Part model, mm, in its own coordinate system. A direction names the side the tool comes from. Round coordinates to 2 decimals unless told otherwise and drop trailing zeros. Write each loop counter-clockwise with the first axis right and the second up, starting at its lowest first coordinate (ties: lowest second). Pieces come first, ordered by that corner, then holes. Notation, with made-up numbers: (-20, 30.5) -> (12, 30.5) arc R7 ccw to (12, 36.5) -> close; hole circle Ø4 at (81, 41.25). An arc over 180 degrees is marked (long way). Return JSON: item names as keys, results as strings. Group by question number.
```python
from build123d import *

# Parameters (mm, degrees)
BASE_FLANGE1_DEPTH = 600
EDGE_FLANGE1_DEPTH = 1200
SKETCH7_R          = 4
CUT_EXTRUDE1_DEPTH = 10


# Sheet-metal steps are written as plain solids
with BuildPart() as part:
    # Sketch1 → Base-Flange1 (new, symmetric)
    with BuildSketch(Plane(origin=(0, 0, 0), x_dir=(0, 0, -1), z_dir=(1, 0, 0))):
        with BuildLine():
            Line((0, 0), (0, -299.494103784))
            ThreePointArc((0, -299.494103784), (0.129412109, -299.911119881), (0.47217601, -300.181606158))
            Line((0.47217601, -300.181606158), (649.872346171, -549.950902374))
            ThreePointArc((649.872346171, -549.950902374), (650.002298395, -549.987621585), (650.136770161, -550))
            Line((650.136770161, -550), (950, -550))
            Line((950, -550), (950, -552))
            Line((950, -552), (650.136717071, -552))
            ThreePointArc((650.136717071, -552), (649.637152182, -551.954006147), (649.154377846, -551.817589676))
            Line((649.154377846, -551.817589676), (-0.245782148, -302.04829737))
            ThreePointArc((-0.245782148, -302.04829737), (-1.519211001, -301.043392746), (-2, -299.494103784))
            Line((-2, -299.494103784), (-2, 0))
            Line((-2, 0), (0, 0))
        make_face()
    extrude(amount=BASE_FLANGE1_DEPTH, both=True)

    # Edge-Flange1 section (across the edge) → Edge-Flange1 (add)
    with BuildSketch(Plane(origin=(600, 0.7366, 2), x_dir=(0, -1, 0), z_dir=(-1, 0, 0))):
        with BuildLine():
            Line((-2, 0.7366), (-2, 33))
            Line((-2, 33), (0, 33))
            Line((0, 33), (0, 0.7366))
            ThreePointArc((0, 0.7366), (0.215745145, 0.215745145), (0.7366, 0))
            Line((0.7366, 0), (0.7366, -2))
            ThreePointArc((0.7366, -2), (-1.198468417, -1.198468417), (-2, 0.7366))
        make_face()
    extrude(amount=EDGE_FLANGE1_DEPTH)

    # Sketch7 → Cut-Extrude1 (cut)
    with BuildSketch(Plane.XZ.offset(-0.7366)):
        with Locations(Location((-550, 18.8683, 0), (0, 0, 270))):
            Circle(SKETCH7_R)
        with Locations(Location((-450, 18.8683, 0), (0, 0, 270))):
            Circle(SKETCH7_R)
        with Locations(Location((-350, 18.8683, 0), (0, 0, 270))):
            Circle(SKETCH7_R)
        with Locations(Location((-250, 18.8683, 0), (0, 0, 270))):
            Circle(SKETCH7_R)
        with Locations(Location((-150, 18.8683, 0), (0, 0, 270))):
            Circle(SKETCH7_R)
        with Locations(Location((-50, 18.8683, 0), (0, 0, 270))):
            Circle(SKETCH7_R)
        with Locations(Location((50, 18.8683, 0), (0, 0, 270))):
            Circle(SKETCH7_R)
        with Locations(Location((150, 18.8683, 0), (0, 0, 270))):
            Circle(SKETCH7_R)
        with Locations(Location((250, 18.8683, 0), (0, 0, 270))):
            Circle(SKETCH7_R)
        with Locations(Location((350, 18.8683, 0), (0, 0, 270))):
            Circle(SKETCH7_R)
        with Locations(Location((450, 18.8683, 0), (0, 0, 270))):
            Circle(SKETCH7_R)
        with Locations(Location((550, 18.8683, 0), (0, 0, 270))):
            Circle(SKETCH7_R)
    extrude(amount=-CUT_EXTRUDE1_DEPTH, mode=Mode.SUBTRACT)


solid = part.part
```
Item 1: Cut at C-C (z = -579). Write the cut outline in (x, y).
Item 2: Cut at B-B (y = -108). Write the cut outline in (x, z).
Item 3: Wall check: L1, parallel to Z at x = -450, y = 1.9; L2, parallel to Y at x = 500.5, z = -877.5; L3, parallel to Z at x = 134, y = -140.5. Give the ranges that are in metal, low to high.
Item 4: Which spindle directions (+Z, -Z, +X, -X, +Y, -Y) get a long thin tool onto all of the face, cutting with end or side? Do faces 1 (the face through (8, 0.737, 19)), 2 (the face through (8, -148, 0)), 3 (the face through (8, 2.737, 19)). Say none if no direction does.
Item 5: Flat gauge pins, fed straight in: P1, Ø5, axis at x = -350, z = 18.87, coming from the -Y side; P2, Ø10.5, axis at x = 350, z = 18.87, coming from the -Y side; P3, Ø12, axis at x = -407, z = -599, coming from the -Y side; P4, Ø6, axis at x = -30, z = -170.5, coming from the +Y side. Where does each tip first touch, or does it go through?
Item 6: Cut at A-A (x = -132). Write the cut outline in (y, z).
Checks:
{
 "1": {"outline": "(-600, -524.84) -> (600, -524.84) -> (600, -522.69) -> (-600, -522.69) -> close"},
 "2": {"outline": "(-600, 0) -> (600, 0) -> (600, 2) -> (-600, 2) -> close"},
 "3": {"L1": "z = 0.77 to 14.87, 22.87 to 35", "L2": "y = -552 to -550", "L3": "z = 0 to 2"},
 "4": {"face 1": "+Z, +X, -X, -Y", "face 2": "-Z, +X, -X, +Y", "face 3": "+Z, -Z, +X, -X, +Y"},
 "5": {"P1": "passes through", "P2": "stops at y = 0.74", "P3": "stops at y = -534.84", "P4": "stops at y = -364.42"},
 "6": {"outline": "(-552, -950) -> (-550, -950) -> (-550, -650.14) arc R0.74 cw to (-549.95, -649.87) -> (-300.18, -0.47) arc R0.74 cw to (-299.49, 0) -> (0, 0) arc R2.74 ccw to (2.74, 2.74) -> (2.74, 35) -> (0.74, 35) -> (0.74, 2.74) arc R0.74 cw to (0, 2) -> (-299.49, 2) arc R2.74 ccw to (-302.05, 0.25) -> (-551.82, -649.15) arc R2.74 ccw to (-552, -650.14) -> close"}
}
